```python
from build123d import *

# Parameters (mm, degrees)
BOSS_EXTRUDE1_DEPTH = 1.5875
SKETCH2_R           = 1.25
CUT_EXTRUDE1_DEPTH  = 2.5875


with BuildPart() as part:
    # Sketch1 → Boss-Extrude1 (new body)
    with BuildSketch(Plane.XY):
        with BuildLine():
            Line((7.96, -9.5), (-7.96, -9.5))
            ThreePointArc((-7.96, -9.5), (-9.756051224, -8.756051224), (-10.5, -6.96))
            Line((-10.5, -6.96), (-10.5, 6.96))
            ThreePointArc((-10.5, 6.96), (-9.756051224, 8.756051224), (-7.96, 9.5))
            Line((-7.96, 9.5), (7.96, 9.5))
            ThreePointArc((7.96, 9.5), (9.756051224, 8.756051224), (10.5, 6.96))
            Line((10.5, 6.96), (10.5, -6.96))
            ThreePointArc((10.5, -6.96), (9.756051224, -8.756051224), (7.96, -9.5))
        make_face()
    extrude(amount=BOSS_EXTRUDE1_DEPTH)

    # Sketch2 → Cut-Extrude1 (cut, through all)
    with BuildSketch(Plane.XY.offset(1.5875)):
        with Locations((-7.96, 6.96)):
            Circle(SKETCH2_R)
        with Locations((7.96, 6.96)):
            Circle(SKETCH2_R)
        with Locations((7.96, -6.96)):
            Circle(SKETCH2_R)
        with Locations((-7.96, -6.96)):
            Circle(SKETCH2_R)
    extrude(amount=-CUT_EXTRUDE1_DEPTH, mode=Mode.SUBTRACT)


solid = part.part
```
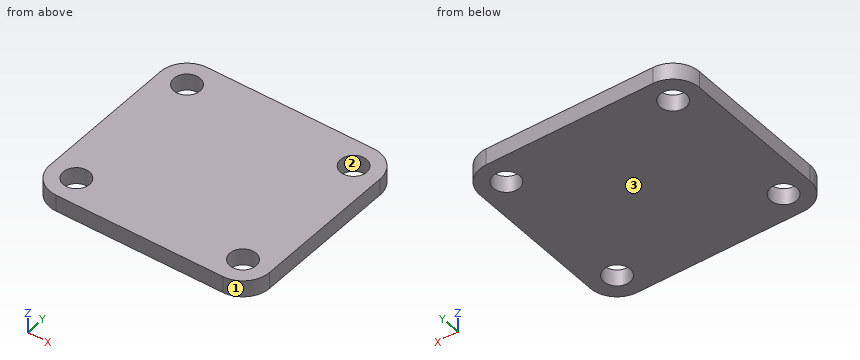
For this review, take the finished solid that the model builds, in its own axes (mm). Face numbers are marked on the shaded views. Coordinates: 2 decimals unless noted, no trailing zeros. Write each loop counter-clockwise with the first axis right and the second up, starting at its lowest first coordinate (ties: lowest second). Pieces come first, ordered by that corner, then holes.
(1) The part is to be moulded in two halves that separate along Y. For the marked faces 1, 2 and 3, say which applies: +Y half, -Y half, draft (parallel to the pull), parting line (faces both ways), or undercut.
(2) Wall thickness on probe 1 along Y at (x, z) = (-8, 0.8); probe 2 along X at (y, z) = (7, 0.8); probe 3 along X at (y, z) = (6, 0.9): over which ranges is each line inside the solid? List them lowest first.
(3) Add section A-A on z = 0.3. Give the boundary of the cut face in (x, y), then the cut area to 3 significant figures.
(4) Add section B-B on y = 7.25. Give the boundary of the cut face in (x, z), then the cut area to 3 significant figures.
(5) For pin 1 Ø1.5 at (x, y) = (7.96, 6.96) entering from -Z, flat-tipped, find the tip position at first contact; note if it passes through.
Answer sheet:
1. face 1: -Y half
1. face 2: undercut
1. face 3: draft
2. probe 1: y = -9.5 to -8.21, -5.71 to 5.71, 8.21 to 9.5
2. probe 2: x = -10.5 to -9.21, -6.71 to 6.71, 9.21 to 10.5
2. probe 3: x = -10.5 to -8.76, -7.16 to 7.16, 8.76 to 10.5
3. outline: (-10.5, -6.96) arc R2.54 ccw to (-7.96, -9.5) - (7.96, -9.5) arc R2.54 ccw to (10.5, -6.96) - (10.5, 6.96) arc R2.54 ccw to (7.96, 9.5) - (-7.96, 9.5) arc R2.54 ccw to (-10.5, 6.96) - close; hole circle Ø2.5 at (-7.96, -6.96); hole circle Ø2.5 at (-7.96, 6.96); hole circle Ø2.5 at (7.96, -6.96); hole circle Ø2.5 at (7.96, 6.96)
3. area: 374 mm2
4. outline: (-10.48, 0) - (-9.18, 0) - (-9.18, 1.59) - (-10.48, 1.59) - close; (-6.74, 0) - (6.74, 0) - (6.74, 1.59) - (-6.74, 1.59) - close; (9.18, 0) - (10.48, 0) - (10.48, 1.59) - (9.18, 1.59) - close
4. area: 25.6 mm2
5. pin 1: passes through
